Geometry check sheet. Reference: the model listing, model coordinates, mm. A direction names the side the tool comes from. Round coordinates to 2 decimals unless told otherwise and drop trailing zeros. Order: outer loops, then holes, each group sorted by start corner. A loop starts at its lowest first (then second) coordinate and runs counter-clockwise, first axis right, second up. Notation, with made-up numbers: (-7, 0) - (42, 0) arc R14 ccw to (42, 10) - close; hole circle Ø3 at (36, 55.5). An arc over 180 degrees is marked (long way). Answer as CSV lines item,"result". Start each with the question number.
```python
from build123d import *

# Parameters (mm, degrees)
PAD002_DEPTH = 15
SKETCH006_R  = 2
PAD003_DEPTH = 1
SKETCH007_W  = 12
SKETCH007_H  = 10
PAD004_DEPTH = 12.5
FILLET_R     = 0.5
SKETCH008_R  = 1.5
PAD005_DEPTH = 10


with BuildPart() as part:
    # Sketch005 → Pad002 (new body)
    with BuildSketch(Plane.YZ):
        with BuildLine():
            ThreePointArc((-3.316625, 5), (-6, 0), (-3.316625, -5))
            Line((-3.316625, -5), (3.316625, -5))
            ThreePointArc((3.316625, -5), (6, 0), (3.316625, 5))
            Line((-3.316625, 5), (3.316625, 5))
        make_face()
    extrude(amount=PAD002_DEPTH)

    # Sketch006 → Pad003 (join)
    with BuildSketch(Plane.YZ):
        Circle(SKETCH006_R)
    extrude(amount=-PAD003_DEPTH)

    # Sketch007 → Pad004 (join)
    with BuildSketch(Plane.YZ.offset(15)):
        Rectangle(SKETCH007_W, SKETCH007_H)
    extrude(amount=PAD004_DEPTH)

    # Fillet
    fillet_edges = [part.edges().sort_by_distance(p)[0] for p in [
        (21.25, -6, 5),
        (21.25, 6, 5),
        (21.25, -6, -5),
        (21.25, 6, -5),
    ]]
    fillet(fillet_edges, radius=FILLET_R)

    # Sketch008 → Pad005 (join)
    with BuildSketch(Plane.YZ.offset(27.5)):
        Circle(SKETCH008_R)
    extrude(amount=PAD005_DEPTH)


with BuildPart() as part_1:
    # Body002 placement: moved
    add(part.part.moved(Location((20, 6, 0))))


solid = part_1.part
```
1. Section check C-C on x = 48. Record the boundary of the cut face in (y, z), plus the area to 3 significant figures.
2. Section check D-D on y = 2. Record the boundary of the cut face in (x, z).
3. Go/stop test with a flat-tipped pin: pin 1 Ø0.8 at (y, z) = (1.5, -1.5) entering from -X. Record where the tip stops, or that it passes through.
4. Access from +Z, -Z, +X, -X, +Y, -Y to the whole of each face (thin tool, end or side, straight path). Record for faces 1 (the face through (27, 0, 0)), 2 (the face through (35, 1, -4)), 3 (the face through (19.5, 4.4, -1.2)), 4 (the face through (47.5, 4.6, -1)), 5 (the face through (35, 1, 4)).
5. Thickness scan on probe 1 along X at (y, z) = (2.5, -4.5); probe 2 along Y at (x, z) = (32.5, 0.5); probe 3 along Y at (x, z) = (33, -3). Record the ranges inside material, lowest first.
6. Section check A-A on y = 6. Record the boundary of the cut face in (x, z).
7. Section check B-B on z = 0.75. Record the boundary of the cut face in (x, y), plus the area to 3 significant figures.
Numbers:
1,outline,"circle Ø3 at (6, 0)"
1,area,"7.07 mm2"
2,outline,"(20, -4.47) - (35, -4.47) - (35, -5) - (47.5, -5) - (47.5, 5) - (35, 5) - (35, 4.47) - (20, 4.47) - close"
3,pin 1,"stops at x = 20"
4,face 1,"-X, -Y"
4,face 2,"-Z, -X, -Y"
4,face 3,"-X"
4,face 4,"+X"
4,face 5,"+Z, -X, -Y"
5,probe 1,"x = 20 to 47.5"
5,probe 2,"y = 0.02 to 11.98"
5,probe 3,"y = 0.8 to 11.2"
6,outline,"(19, -2) - (20, -2) - (20, -5) - (47.5, -5) - (47.5, -1.5) - (57.5, -1.5) - (57.5, 1.5) - (47.5, 1.5) - (47.5, 5) - (20, 5) - (20, 2) - (19, 2) - close"
7,outline,"(19, 4.15) - (20, 4.15) - (20, 0.05) - (35, 0.05) - (35, 0) - (47.5, 0) - (47.5, 4.7) - (57.5, 4.7) - (57.5, 7.3) - (47.5, 7.3) - (47.5, 12) - (35, 12) - (35, 11.95) - (20, 11.95) - (20, 7.85) - (19, 7.85) - close"
7,area,"358 mm2"
